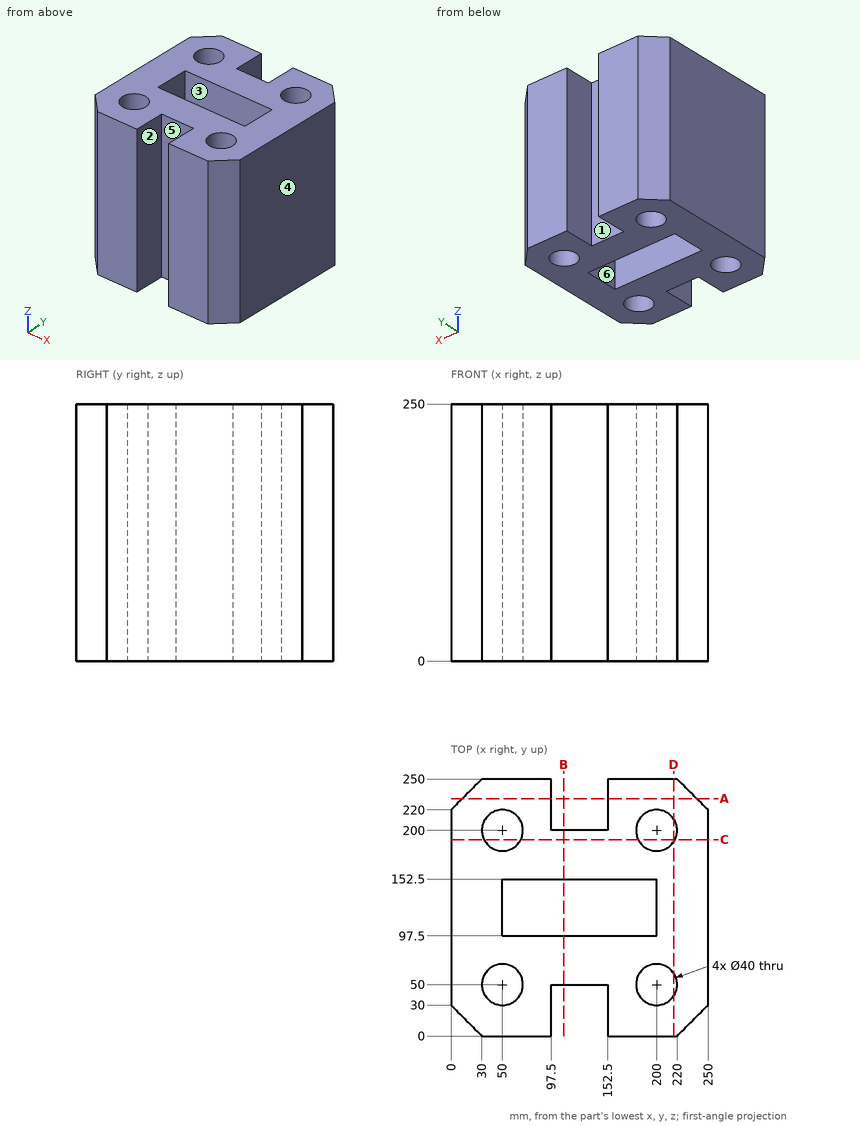
Geometry: see drawing. Coordinates: mm, zero at the bounding-box minimum. A direction names the side the tool comes from. Give positions to 0.01 mm unless a question says otherwise; leave off trailing zeros. Loops run counter-clockwise (first coordinate to the right, second up) from the corner with the lowest first, then second, coordinate; pieces in that order, holes last. Notation, with made-up numbers: (15.25, 7.5) -> (37.25, 7.5) arc R34 ccw to (37.25, 40.5) -> close; hole circle Ø1 at (10.25, 81.25). An arc over 180 degrees is marked (long way). Answer as a JSON object with one key per item and string values. Group by question number.
Item 1: Line query: probe 1 along X at (y, z) = (134, 202); probe 2 along X at (y, z) = (49.5, 93.5); probe 3 along Y at (x, z) = (39, 51). Output: solid intervals per line, ascending.
Item 2: Pull-direction query (Y, two-part tool) for the marked faces 4, 5 and 6; classes: released by +Y, released by -Y, zero draft, split by the parting line, or undercut.
Item 3: Reachability of the marked faces 1, 2 and 3 from +Z, -Z, +X, -X, +Y, -Y: full face, straight path, thin tool, end or side. Return the list, or none.
Item 4: Cut plane C-C, the plane y = 191. Return the cut outline in (x, z).
Item 5: Cut plane A-A, the plane y = 231. Return the cut outline in (x, z).
Item 6: Pin query (flat end, axial travel): P1, Ø15, axis at y = 237, z = 94, coming from the +X side; P2, Ø5, axis at y = 224.5, z = 69, coming from the +X side. Return the tip coordinate at first contact, or that it passes through.
Item 7: Cut plane D-D, the plane x = 216.5. Return the cut outline in (y, z).
Item 8: Cut plane B-B, the plane x = 109.5. Return the cut outline in (y, z), and give its area (4 significant figures).
Checks:
{
 "1": {"probe 1": "x = 0 to 50, 200 to 250", "probe 2": "x = 0 to 30.01, 69.99 to 97.5, 152.5 to 180.01, 219.99 to 250", "probe 3": "y = 0 to 33.3, 66.7 to 183.3, 216.7 to 250"},
 "2": {"face 4": "zero draft", "face 5": "released by -Y", "face 6": "undercut"},
 "3": {"face 1": "+Z, -Z, +Y", "face 2": "+Z, -Z, -Y", "face 3": "+Z, -Z"},
 "4": {"outline": "(0, 0) -> (32.14, 0) -> (32.14, 250) -> (0, 250) -> close; (67.86, 0) -> (182.14, 0) -> (182.14, 250) -> (67.86, 250) -> close; (217.86, 0) -> (250, 0) -> (250, 250) -> (217.86, 250) -> close"},
 "5": {"outline": "(11, 0) -> (97.5, 0) -> (97.5, 250) -> (11, 250) -> close; (152.5, 0) -> (239, 0) -> (239, 250) -> (152.5, 250) -> close"},
 "6": {"P1": "stops at x = 240.5", "P2": "stops at x = 248"},
 "7": {"outline": "(0, 0) -> (38.7, 0) -> (38.7, 250) -> (0, 250) -> close; (61.3, 0) -> (188.7, 0) -> (188.7, 250) -> (61.3, 250) -> close; (211.3, 0) -> (250, 0) -> (250, 250) -> (211.3, 250) -> close"},
 "8": {"outline": "(50, 0) -> (97.5, 0) -> (97.5, 250) -> (50, 250) -> close; (152.5, 0) -> (200, 0) -> (200, 250) -> (152.5, 250) -> close", "area": "23,750 mm²"}
}
